Verification items for the finished model (mm, model axes). Round coordinates to 2 decimals unless told otherwise and drop trailing zeros. Write each loop counter-clockwise with the first axis right and the second up, starting at its lowest first coordinate (ties: lowest second). Pieces come first, ordered by that corner, then holes. Notation, with made-up numbers: M -26.75,-18 L 23.25,-18 A14 cw 23.25,7 Z; hole C -10,-31 d5. An arc over 180 degrees is marked long. Use a Markdown table: item, result. Add a question column.
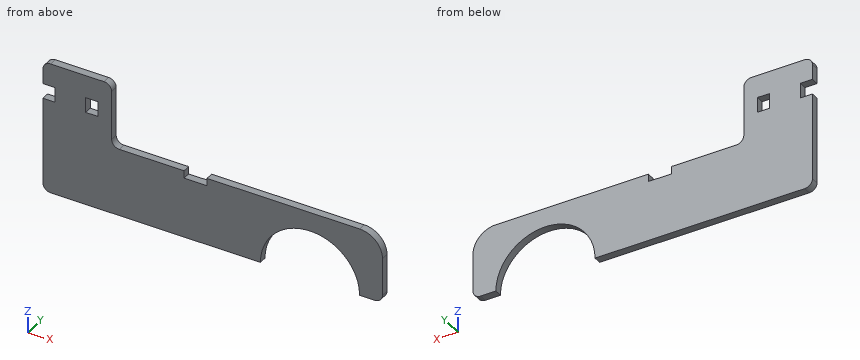
from build123d import *

# Parameters (mm, degrees)
F0_W     = 8
F0_H     = 10
F1_DEPTH = 5


with BuildPart() as f1:
    # F0 (on Front) → F1 (new body)
    with BuildSketch(Plane.XZ):
        with BuildLine():
            ThreePointArc((-32.5, 0), (0, 32.5), (32.5, 0))
            Line((32.5, 0), (42.5, 0))
            ThreePointArc((42.5, 0), (46.035534, 1.464466), (47.5, 5))
            Line((47.5, 5), (47.5, 30))
            ThreePointArc((47.5, 30), (43.106602, 40.606602), (32.5, 45))
            Line((32.5, 45), (-67.5, 45))
            Line((-67.5, 45), (-67.5, 40))
            Line((-67.5, 40), (-82.5, 40))
            Line((-82.5, 40), (-82.5, 45))
            Line((-82.5, 45), (-125, 45))
            ThreePointArc((-125, 45), (-128.535534, 46.464466), (-130, 50))
            Line((-130, 50), (-130, 82.5))
            ThreePointArc((-130, 82.5), (-131.464466, 86.035534), (-135, 87.5))
            Line((-135, 87.5), (-170, 87.5))
            ThreePointArc((-170, 87.5), (-173.535534, 86.035534), (-175, 82.5))
            Line((-175, 82.5), (-175, 72.5))
            Line((-175, 72.5), (-167, 72.5))
            Line((-167, 72.5), (-167, 62.5))
            Line((-167, 62.5), (-175, 62.5))
            Line((-175, 62.5), (-175, 5))
            ThreePointArc((-175, 5), (-173.535534, 1.464466), (-170, 0))
            Line((-170, 0), (-32.5, 0))
        make_face()
        with Locations((-143, 67.5)):
            Rectangle(F0_W, F0_H, mode=Mode.SUBTRACT)
    extrude(amount=F1_DEPTH)


solid = f1.part
1. Scan lines: line 1 along X through (y, z) = (-1.65, 71.5); line 2 along X through (y, z) = (-0.8, 59); line 3 along X through (y, z) = (-3, 30). Record each from-to range of solid material in increasing order. Write a range as from..to.
2. Cross-section at C-C on z = 28. Enter the section's corners in (x, y), plus the area to 4 significant figures.
3. Cross-section at B-B on y = -2.8. Enter the section's corners in (x, z), plus the area to 3 significant figures.
4. Cross-section at D-D on x = -105. Enter the section's corners in (y, z), plus the area to 3 significant figures.
5. Cross-section at A-A on z = 69. Enter the section's corners in (x, y).
6. Depth check by flat-ended pin: pin 1 Ø1 at (x, y) = (-43, -3) entering from +Z; pin 2 Ø2.5 at (x, y) = (-75.5, -2) entering from +Z; pin 3 Ø2.5 at (y, z) = (-3, 42.5) entering from +X. Enter the tip coordinate at first touch or a pass-through.
Answer:
| question | item | result |
|---|---|---|
| 1 | line 1 | x = -167..-147, -139..-130 |
| 1 | line 2 | x = -175..-130 |
| 1 | line 3 | x = -175..-12.5, 12.5..47.5 |
| 2 | outline | M -175,-5 L -16.5,-5 L -16.5,0 L -175,0 Z; M 16.5,-5 L 47.5,-5 L 47.5,0 L 16.5,0 Z |
| 2 | area | 947.5 mm^2 |
| 3 | outline | M -175,5 A5 ccw -170,0 L -32.5,0 A32.5 cw 32.5,0 L 42.5,0 A5 ccw 47.5,5 L 47.5,30 A15 ccw 32.5,45 L -67.5,45 L -67.5,40 L -82.5,40 L -82.5,45 L -125,45 A5 cw -130,50 L -130,82.5 A5 ccw -135,87.5 L -170,87.5 A5 ccw -175,82.5 L -175,72.5 L -167,72.5 L -167,62.5 L -175,62.5 Z; hole M -147,62.5 L -139,62.5 L -139,72.5 L -147,72.5 Z |
| 3 | area | 9,970 mm^2 |
| 4 | outline | M -5,0 L 0,0 L 0,45 L -5,45 Z |
| 4 | area | 225 mm^2 |
| 5 | outline | M -167,-5 L -147,-5 L -147,0 L -167,0 Z; M -139,-5 L -130,-5 L -130,0 L -139,0 Z |
| 6 | pin 1 | stops at z = 45 |
| 6 | pin 2 | stops at z = 40 |
| 6 | pin 3 | stops at x = 42.42 |
